The model under review builds one solid part; all positions refer to its coordinate system, in mm. Face numbers are marked on the shaded views. A direction names the side the tool comes from. Coordinates: 2 decimals unless noted, no trailing zeros. Order: outer loops, then holes, each group sorted by start corner. A loop starts at its lowest first (then second) coordinate and runs counter-clockwise, first axis right, second up. Notation, with made-up numbers: (9.5, 68) -> (68.5, 68) arc R27 ccw to (68.5, 87) -> close; hole circle Ø8 at (2, 57). An arc over 180 degrees is marked (long way). Put each result on its own line as item: value.
from build123d import *

# Parameters (mm, degrees)
F0_W      = 260.35
F0_H      = 28.575
F1_FACE_R = 28.575
F3_DEPTH  = 38.1
F4_SIZE   = 5.08


with BuildPart() as f1:
    # F0 (on Front) → F1 (revolve)
    with BuildSketch(Plane.XZ):
        with Locations((-130.175, 14.2875)):
            Rectangle(F0_W, F0_H)
    revolve(axis=Axis((-130.175, 0, 0), (-1, 0, 0)))

    # F2 (on Right) + F1_face (on face) → F3 (join)
    with BuildSketch(Plane.YZ):
        Polygon((-39.6875, -22.913589), (0, -45.827178), (39.6875, -22.913589), (39.6875, 22.913589), (0, 45.827178), (-39.6875, 22.913589), align=None)
    with BuildSketch(Plane.YZ):
        Circle(F1_FACE_R)
    extrude(amount=F3_DEPTH)

    # F4
    f4_edges = [f1.edges().sort_by_distance(p)[0] for p in [
        (-260.35, 0, -28.575),
    ]]
    chamfer(f4_edges, length=F4_SIZE)


solid = f1.part
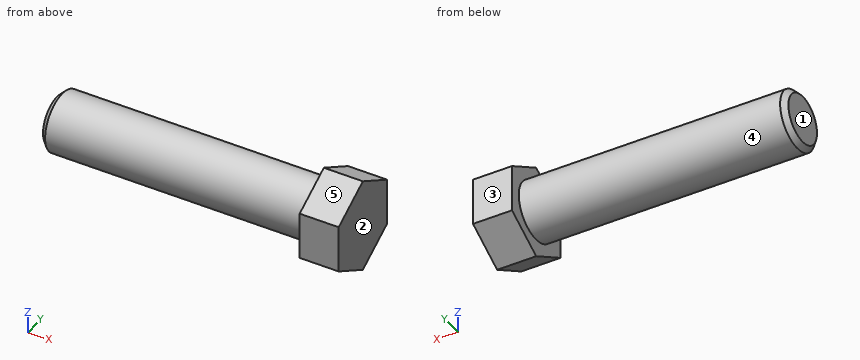
Item 1: Mouldability with a two-part tool opening along X and no side actions: class the marked faces 1, 2 and 3 as +X half, -X half, draft (parallel to the pull), parting line (faces both ways), or undercut.
Answers below:
face 1: -X half
face 2: +X half
face 3: draft
Item 2: Consider section B-B on x = -66. Write out the cut boundary in (y, z) (3 decimals), and give its area (3 significant figures).
Answers below:
outline: circle Ø57.15 at (0, 0)
area: 2,570 mm^2
Item 3: Consider section C-C on z = 32.5. Write out the cut boundary in (x, y).
Answers below:
outline: (0, -23.08) -> (38.1, -23.08) -> (38.1, 23.08) -> (0, 23.08) -> close
Item 4: For the marked faces 4 and 5, list the 3-axis set-ups (+Z, -Z, +X, -X, +Y, -Y) from which the entire face can be reached by the end or side of a thin tool; tool diameter is ignored.
Answers below:
face 4: -X
face 5: +Z, +X, -X, -Y
Item 5: For pin 1 Ø6 at (x, y) = (-6, -21.5) entering from +Z; pin 2 Ø8 at (x, z) = (-65.5, -15.5) entering from +Y; pin 3 Ø8 at (x, y) = (-19.5, 10.5) entering from -Z, all flat-tipped, find the tip position at first contact; note any pin that passes through.
Answers below:
pin 1: z = 21.78
pin 2: y = 26.16
pin 3: z = -27.83
Item 6: For line 1 (X direction, y = 32, z = -18.5); line 2 (Z direction, x = -245, y = 17); line 3 (Z direction, x = -232, y = -17.5), list the stretches that pass through material, from the lowest coordinate up. Write a range as from..to.
Answers below:
line 1: 0..38.1
line 2: -22.97..22.97
line 3: -22.59..22.59
